```python
from build123d import *

# Parameters (mm, degrees)
SKETCH1_W            = 12.7
SKETCH1_H            = 29
BOSS_EXTRUDE1_DEPTH  = 7
HOLE1_D              = 5.6
HOLE1_CBORE_D        = 6
HOLE1_CBORE_DEPTH    = 6
SKETCH4_W            = 29
SKETCH4_H            = 10
BOSS_EXTRUDE2_DEPTH  = 12.7
CUT_EXTRUDE1_DEPTH   = 35.209976615
M3_CLEARANCE_HOLE1_D = 3.6
CHAMFER1_SIZE        = 6
CHAMFER1_SIZE_2      = 0.2


with BuildPart() as part:
    # Sketch1 → Boss-Extrude1 (new body)
    with BuildSketch(Plane(origin=(0, 0, 0), x_dir=(1, 0, 0), z_dir=(0, 1, 0))):
        Rectangle(SKETCH1_W, SKETCH1_H)
    extrude(amount=BOSS_EXTRUDE1_DEPTH)

    # Hole1 (through all)
    with Locations(Plane(origin=(0, 0, 0), x_dir=(-1, 0, 0), z_dir=(0, -1, 0))):
        with Locations((0, -7.5), (0, 7.5)):
            CounterBoreHole(HOLE1_D / 2, HOLE1_CBORE_D / 2, HOLE1_CBORE_DEPTH)

    # Sketch4 → Boss-Extrude2 (add)
    with BuildSketch(Plane.ZY.offset(6.35)):
        with Locations((0, 12)):
            Rectangle(SKETCH4_W, SKETCH4_H)
    extrude(amount=-BOSS_EXTRUDE2_DEPTH)

    # Sketch5 → Cut-Extrude1 (cut, through all)
    with BuildSketch(Plane(origin=(0, 0, -14.5), x_dir=(-1, 0, 0), z_dir=(0, 0, -1))):
        with BuildLine():
            Line((-0.4, 11), (-0.4, 10))
            ThreePointArc((-0.4, 10), (0, 8.293774225), (0.4, 10))
            Line((0.4, 10), (0.4, 11))
            Line((0.4, 11), (2.5, 11))
            Line((2.5, 11), (2.5, 17))
            Line((2.5, 17), (-2.5, 17))
            Line((-2.5, 17), (-2.5, 11))
            Line((-2.5, 11), (-0.4, 11))
        make_face()
    extrude(amount=-CUT_EXTRUDE1_DEPTH, mode=Mode.SUBTRACT)

    # M3 Clearance Hole1 (through all)
    with Locations(Plane.ZY.offset(6.35)):
        with Locations((0, 14)):
            Hole(M3_CLEARANCE_HOLE1_D / 2)

    # Chamfer1
    # the kernel refuses this chamfer: 6, 0.2 mm, written as the material it adds along each edge
    with BuildSketch(Plane(origin=(0, 6, -7.5), x_dir=(-1, 0, 0), z_dir=(0, 0, 1))) as chamfer1_piece_1_section:
        Polygon((3, CHAMFER1_SIZE), (3 - CHAMFER1_SIZE_2, 0), (3, 0), align=None)
    chamfer1_piece_1 = revolve(axis=Axis((0, 6, -7.5), (0, -1, 0)), mode=Mode.PRIVATE)
    chamfer1_piece_1 = split(chamfer1_piece_1, bisect_by=Plane(origin=(2.92947192, 0, -7.5), z_dir=(0, 1, 0)), keep=Keep.TOP, mode=Mode.PRIVATE)
    chamfer1_piece_1 = chamfer1_piece_1 - Plane(origin=(0, 3.000982397, -7.5), x_dir=(1, 0, 0), z_dir=(0, 1, 0)) * Cylinder(2.8, 24, mode=Mode.PRIVATE)
    add(chamfer1_piece_1)
    with BuildSketch(Plane(origin=(0, 6, 7.5), x_dir=(-1, 0, 0), z_dir=(0, 0, 1))) as chamfer1_piece_2_section:
        Polygon((3, CHAMFER1_SIZE), (3 - CHAMFER1_SIZE_2, 0), (3, 0), align=None)
    chamfer1_piece_2 = revolve(axis=Axis((0, 6, 7.5), (0, -1, 0)), mode=Mode.PRIVATE)
    chamfer1_piece_2 = split(chamfer1_piece_2, bisect_by=Plane(origin=(2.92947192, 0, 7.5), z_dir=(0, 1, 0)), keep=Keep.TOP, mode=Mode.PRIVATE)
    chamfer1_piece_2 = chamfer1_piece_2 - Plane(origin=(0, 3.000982397, 7.5), x_dir=(1, 0, 0), z_dir=(0, 1, 0)) * Cylinder(2.8, 24, mode=Mode.PRIVATE)
    add(chamfer1_piece_2)


solid = part.part
```
Geometry check sheet. Reference: the model listing, model coordinates, mm. A direction names the side the tool comes from. Give positions to 0.01 mm unless a question says otherwise; leave off trailing zeros. Order: outer loops, then holes, each group sorted by start corner. A loop starts at its lowest first (then second) coordinate and runs counter-clockwise, first axis right, second up.
1. Section check A-A, the plane z = 0. Enter the section's corners in (x, y).
2. Gauge pin test, flat ends, axial feed: pin 1 Ø1.7 at (x, z) = (-0.5, -9) entering from -Y; pin 2 Ø0.6 at (x, z) = (-2, -1.5) entering from +Y; pin 3 Ø1.1 at (x, y) = (0, 9.19) entering from -Z. Record the tip position at first contact, or that the pin passes through.
3. Section check D-D, the plane z = -7.5. Enter the section's corners in (x, y), and give its area (3 significant figures).
4. Section check B-B, the plane x = 3.5. Enter the section's corners in (y, z), and give its area (3 significant figures).
5. Release check for a two-part mould opening along Y. For faces 1 (the face through (0, 6, 14.5)), 2 (the face through (4.452, 15.785, 0.234)), 3 (the face through (4, 17, 0)) record: pulls with the +Y half, pulls with the -Y half, needs draft (parallel to the pull), parting line crosses it, or undercut.
6. Section check C-C, the plane y = 14. Enter the section's corners in (x, z), and give its area (3 significant figures).
7. Thickness scan on L1, parallel to Z at x = 0, y = 6.4; L2, parallel to X at y = 15, z = 8.75; L3, parallel to Z at x = -1.5, y = 3.5. Record the ranges inside material, lowest first.
8. Access from +Z, -Z, +X, -X, +Y, -Y to the whole of each face (thin tool, end or side, straight path). Record for faces 4 (the face through (-0.607, 6.507, 10.233)), 5 (the face through (-4, 17, 0)), 6 (the face through (-1, 11, 0)).
Values follow:
1. outline: (-6.35, 0) - (6.35, 0) - (6.35, 12.2) - (2.5, 12.2) - (2.5, 11) - (0.4, 11) - (0.4, 10) arc R0.9 cw (long way) to (-0.4, 10) - (-0.4, 11) - (-2.5, 11) - (-2.5, 12.2) - (-6.35, 12.2) - close; (-6.35, 15.8) - (-2.5, 15.8) - (-2.5, 17) - (-6.35, 17) - close; (2.5, 15.8) - (6.35, 15.8) - (6.35, 17) - (2.5, 17) - close
2. pin 1: stops at y = 7
2. pin 2: stops at y = 11
2. pin 3: passes through
3. outline: (-6.35, 0) - (-3, 0) - (-2.8, 6) - (-2.8, 7) - (2.8, 7) - (2.8, 6) - (3, 0) - (6.35, 0) - (6.35, 17) - (2.5, 17) - (2.5, 11) - (0.4, 11) - (0.4, 10) arc R0.9 cw (long way) to (-0.4, 10) - (-0.4, 11) - (-2.5, 11) - (-2.5, 17) - (-6.35, 17) - close
3. area: 142 mm2
4. outline: (0, -14.5) - (17, -14.5) - (17, 14.5) - (0, 14.5) - close; hole circle Ø3.6 at (14, 0)
4. area: 483 mm2
5. face 1: needs draft
5. face 2: undercut
5. face 3: pulls with the +Y half
6. outline: (-6.35, -14.5) - (-2.5, -14.5) - (-2.5, -1.8) - (-6.35, -1.8) - close; (-6.35, 1.8) - (-2.5, 1.8) - (-2.5, 14.5) - (-6.35, 14.5) - close; (2.5, -14.5) - (6.35, -14.5) - (6.35, -1.8) - (2.5, -1.8) - close; (2.5, 1.8) - (6.35, 1.8) - (6.35, 14.5) - (2.5, 14.5) - close
6. area: 196 mm2
7. L1: z = -14.5 to -10.3, -4.7 to 4.7, 10.3 to 14.5
7. L2: x = -6.35 to -2.5, 2.5 to 6.35
7. L3: z = -14.5 to -9.96, -5.04 to 5.04, 9.96 to 14.5
8. face 4: -Y
8. face 5: +Z, -Z, +X, -X, +Y
8. face 6: +Z, -Z, +Y
